Here's the drawing with two shaded views (mm, measured from the low corner). I have some questions. Round coordinates to 2 decimals unless told otherwise and drop trailing zeros. Loops run counter-clockwise (first coordinate to the right, second up) from the corner with the lowest first, then second, coordinate; pieces in that order, holes last.
(1) If I drill on line 1 along X through (y, z) = (2.5, 2.6) (1 decimal); line 2 along Y through (x, z) = (25.4, 2.5); line 3 along Y through (x, z) = (53, 1.25) (1 decimal), over which ranges is the centre line in solid material (lowest first)?
(2) I want a section at B-B on y = 11.43. Give the number of separate pieces and of enclosed holes in the cut face.
(3) I want a section at D-D on x = 25.4. Write out the boundary of the cut face in (y, z) (1 decimal).
(4) I want a section at A-A on x = 40.64. Write out the boundary of the cut face in (y, z) (1 decimal).
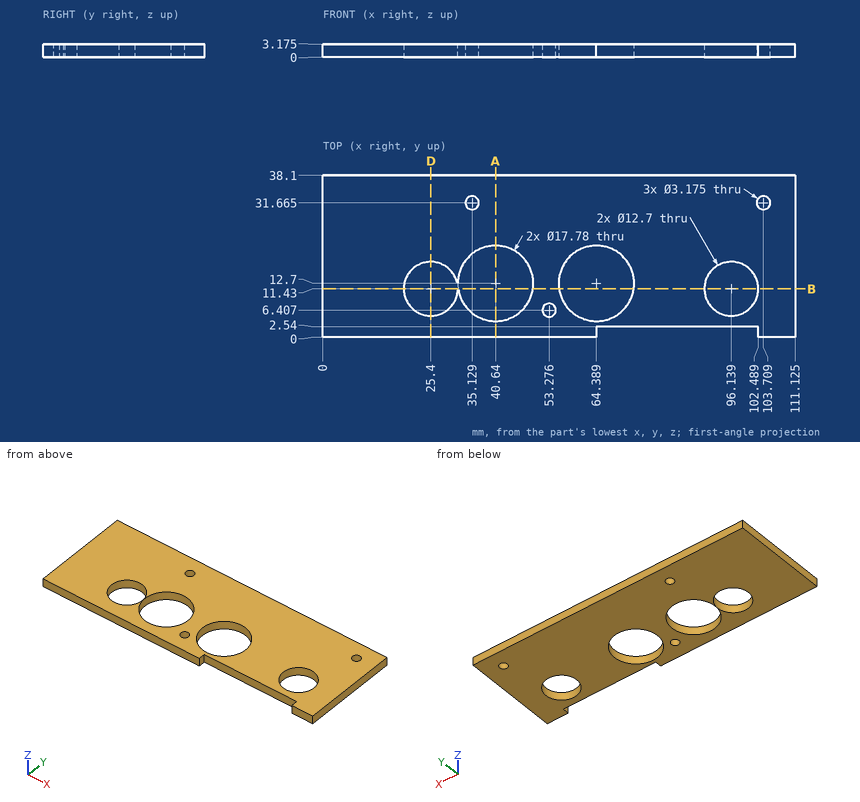
Filled sheet:
1. line 1: x = 0 to 64.4, 102.5 to 111.1
1. line 2: y = 0 to 5.08, 17.78 to 38.1
1. line 3: y = 0 to 4.8, 8 to 38.1
2. separate pieces: 5
2. enclosed holes: 0
3. outline: (0, 0) - (5.1, 0) - (5.1, 3.2) - (0, 3.2) - close; (17.8, 0) - (38.1, 0) - (38.1, 3.2) - (17.8, 3.2) - close
4. outline: (0, 0) - (3.8, 0) - (3.8, 3.2) - (0, 3.2) - close; (21.6, 0) - (38.1, 0) - (38.1, 3.2) - (21.6, 3.2) - close
